Read the model definition and answer for the solid it produces. Units are mm, in the model's axes. A direction names the side the tool comes from. Coordinates: 2 decimals unless noted, no trailing zeros. Loops run counter-clockwise (first coordinate to the right, second up) from the corner with the lowest first, then second, coordinate; pieces in that order, holes last.
Autodesk Inventor part; units mm, degrees
ref_plane "YZ Plane" through (0, 0, 0) normal (1, 0, 0) x (0, 1, 0)
ref_plane "XZ Plane" through (0, 0, 0) normal (0, 1, 0) x (-1, 0, 0)
ref_plane "XY Plane" through (0, 0, 0) normal (0, 0, 1) x (1, 0, 0)
sketch "Sketch1" plane through (0, 0, 0) normal (1, 0, 0) x (0, 1, 0)
  point P0 (0, 0)
sketch "Sketch2" plane through (0, 0, 0) normal (1, 0, 0) x (0, 1, 0)
  line L0 (7, 8.85) -> (-7, 8.85)
  line L1 (-7, 8.85) -> (-7, -8.85)
  line L2 (-7, -8.85) -> (7, -8.85)
  line L3 (7, -8.85) -> (7, 8.85)
  point P0 (0, 0)
  dimension "d0" = 17.7
  dimension "d1" = 14
  dimension "d2" = 8.85
  dimension "d3" = 7
extrude "Extrusion1" add sketch "Sketch2" along normal blind 14
fillet "Fillet1" radius 2 2 edges at (7, 7, 8.85) (7, 7, -8.85)
sketch "Sketch5" plane through (14, 0, 0) normal (1, 0, 0) x (0, 0, -1)
  line L0 (-7.35, 6) -> (7.35, 6)
  line L1 (7.35, 6) -> (7.35, -7)
  line L2 (7.35, -7) -> (-7.35, -7)
  line L3 (-7.35, -7) -> (-7.35, 6)
  line L4 (6.85, 7) -> (-6.85, 7)
  line L5 (8.85, -7) -> (8.85, 5)
  line L6 (-8.85, -7) -> (8.85, -7)
  line L7 (-8.85, 5) -> (-8.85, -7)
  point P0 (0, 0)
  dimension "d19" = 1
  dimension "d20" = 1.5
  dimension "d21" = 0
  dimension "d22" = 1.5
extrude "Extrusion2" cut sketch "Sketch5" against normal blind 2
fillet "Fillet2" radius 1 1 edges at (13, 6, 7.35)
fillet "Fillet3" radius 1 1 edges at (13, 6, -7.35)
sketch "Sketch6" plane through (12, 0, 0) normal (1, 0, 0) x (0, 0, -1)
  line L0 (-3.75, 5.3) -> (3.75, 5.3)
  line L1 (3.75, 5.3) -> (3.75, -4.4)
  line L2 (3.75, -4.4) -> (-3.75, -4.4)
  line L3 (-3.75, -4.4) -> (-3.75, 5.3)
  line L4 (-6.35, 6) -> (6.35, 6)
  line L5 (7.35, -7) -> (-7.35, -7)
  line L6 (-7.35, -7) -> (-7.35, 5)
  line L7 (7.35, 5) -> (7.35, -7)
  point P0 (0, 0)
  dimension "d27" = 9.7
  dimension "d28" = 7.5
  dimension "d35" = 0.7
  dimension "d36" = 2.6
  dimension "d107" = 3.75
extrude "Extrusion3" cut sketch "Sketch6" against normal blind 2
ref_plane "Work Plane2" through (7, 0, 0) normal (1, 0, 0) x (0, 0, -1)
mirror "Mirror1" about plane through (7, 0, 0) normal (1, 0, 0) of "Extrusion2"
sketch "Sketch11" plane through (2, -7, -7.35) normal (-1, 0, 0) x (0, 0, 1)
  line L0 (4.45, 2) -> (10.25, 2)
  line L1 (10.25, 2) -> (10.25, 6.7)
  line L2 (10.25, 6.7) -> (4.45, 6.7)
  line L3 (4.45, 6.7) -> (4.45, 2)
  line L4 (10.725, 6.7) -> (3.975, 6.7)
  line L5 (3.975, 6.7) -> (3.975, 10)
  line L6 (3.975, 10) -> (10.725, 10)
  line L7 (10.725, 10) -> (10.725, 6.7)
  line L8 (14.7, 0) -> (0, 0)
  point P0 (7.35, 7)
  point P1 (10.25, 6.7)
  dimension "d52" = 5.8
  dimension "d53" = 4.7
  dimension "d54" = 2
  dimension "d55" = 3.3
  dimension "d56" = 6.75
  dimension "d57" = 2.9
  dimension "d58" = 3.375
extrude "Extrusion5" cut sketch "Sketch11" against normal blind 3.3
fillet "Fillet4" radius 0.001 2 edges at (3.65, 3, -3.375) (3.65, 3, 3.375)
fillet "Fillet5" radius 0.001 2 edges at (3.65, -0.3, -3.375) (3.65, -0.3, 3.375)
fillet "Fillet6" radius 1 1 edges at (1, 6, 7.35)
fillet "Fillet7" radius 1 1 edges at (1, 6, -7.35)
sketch "Sketch15" plane through (0, -7, -8.85) normal (0, -1, 0) x (1, 0, 0)
  line L0 (0, 2) -> (14, 2)
  circle A0 centre (4, 2) radius 0.5
  line L1 (0, 1.5) -> (0, 0)
  line L2 (12, 1.5) -> (12, 16.2)
  line L3 (2, 16.2) -> (2, 1.5)
  line L4 (7, 21.24) -> (7, -3.54)
  point P0 (0, 8.85)
  point P1 (12, 3.75)
  point P2 (2, 3.35)
  dimension "d74" = 1
  dimension "d120" = 4
extrude "Extrusion8" add sketch "Sketch15" along normal blind 4
mirror "Mirror3" about plane through (0, 0, 0) normal (0, 0, 1) of "Extrusion8"
mirror "Mirror4" about plane through (7, 0, 0) normal (1, 0, 0) of "Extrusion8", "Mirror3"
sketch "Sketch18" plane through (2, 3, -3.374) normal (0, -1, 0) x (1, 0, 0)
  line L0 (3.3, -0.001) -> (0, -0.001)
  line L1 (0, -0.001) -> (0, 6.749)
  line L2 (0, 6.749) -> (3.3, 6.749)
  line L3 (3.3, 6.749) -> (3.3, -0.001)
  line L4 (0, -0.001) -> (3.3, -0.001)
  line L5 (3.3, 6.749) -> (0, 6.749)
  line L6 (0, 0) -> (0, 6.748)
  line L7 (3.3, 0) -> (3.3, 6.748)
  point P0 (-2, 3.374)
extrude "Extrusion9" cut sketch "Sketch18" against normal through all
sketch "Sketch19" plane through (0, -7, 8.85) normal (0, -1, 0) x (1, 0, 0)
  line L0 (13, -0.8) -> (12, -0.8)
  line L1 (12, -0.8) -> (12, -1.5)
  line L2 (12, -1.5) -> (13, -1.5)
  line L3 (13, -1.5) -> (13, -0.8)
  point P0 (0, -8.85)
  dimension "d103" = 0.7
  dimension "d104" = 1
sketch3d "3D Sketch3"
  line L0 (14, -7, 7.35) -> (14, 5, 7.35)
  arc A0 (14, 5, 7.35) -> (14, 6, 6.35) centre (14, 5, 6.35) ccw
  line L1 (14, 6, 6.35) -> (14, 6, -6.35)
  arc A1 (14, 6, -6.35) -> (14, 5, -7.35) centre (14, 5, -6.35) ccw
  line L2 (14, 5, -7.35) -> (14, -7, -7.35)
sweep "Sweep3" cut profiles "Sketch19" path "3D Sketch3"
mirror "Mirror6" about plane through (7, 0, 0) normal (1, 0, 0) of "Sweep3"
sketch "Sketch20" plane through (12, 0, 0) normal (1, 0, 0) x (0, 0, -1)
  line L0 (-2.9, -5) -> (2.9, -5)
  line L1 (2.9, -5) -> (2.9, -7)
  line L2 (2.9, -7) -> (-2.9, -7)
  line L3 (-2.9, -7) -> (-2.9, -5)
  line L4 (3.6, 4.6) -> (3.6, -4.3)
  line L5 (-3.6, -4.3) -> (-3.6, 5.3)
  line L6 (3.6, -4.3) -> (-3.6, -4.3)
  line L7 (5.45, -7) -> (-5.45, -7)
  point P0 (0, 0)
  dimension "d109" = 0.7
  dimension "d110" = 0.7
  dimension "d116" = 2
extrude "Extrusion10" cut sketch "Sketch20" against normal through all
sketch "Sketch21" plane through (12, 0, 0) normal (1, 0, 0) x (0, 0, -1)
  line L0 (-2.9, -4.4) -> (2.9, -4.4)
  line L1 (2.9, -4.4) -> (2.9, -5)
  line L2 (2.9, -5) -> (-2.9, -5)
  line L3 (-2.9, -5) -> (-2.9, -4.4)
  line L4 (3.75, -4.4) -> (-3.75, -4.4)
  line L5 (-2.9, -5) -> (2.9, -5)
  line L6 (2.9, -5) -> (2.9, -7)
  line L7 (-2.9, -7) -> (-2.9, -5)
  point P0 (0, 0)
extrude "Extrusion11" cut sketch "Sketch21" against normal blind 2
properties part number "fingertip skeleton 5"
Item 1: Find the intervals of material crossed by line 1 along Y through (x, z) = (10.75, 3.5); line 2 along X through (y, z) = (6.25, -0.75); line 3 along X through (y, z) = (2, 8), in increasing order.
Numbers:
line 1: y = -7 to -4.4, 5.3 to 7
line 2: x = 0 to 1, 5.3 to 12, 13 to 14
line 3: x = 0 to 1, 2 to 12, 13 to 14
Item 2: Determine the mould class of faces 5 (the face through (3.892, -8.972, -6.362)), 6 (the face through (7, -1, -8.85)) for opening direction X: released by +X, released by -X, zero draft, split by the parting line, or undercut.
Numbers:
face 5: undercut
face 6: zero draft
Item 3: A cutting plane is placed at C-C on z = 4.75. Determine the outline of the cut face in (x, y), then the cut area to 3 significant figures.
Numbers:
outline: (0, 6) - (1, 6) - (1, 6.7) - (2, 6.7) - (2, -7) - (12, -7) - (12, 6.7) - (13, 6.7) - (13, 6) - (14, 6) - (14, 7) - (0, 7) - close
area: 143 mm2
Item 4: Which of the six approach directions +Z, -Z, +X, -X, +Y, -Y give full straight-line access (tool end or side, diameter ignored) to faces 1 (the face through (4, 5, 3.375)), 2 (the face through (13.493, 5.715, -7.049)), 3 (the face through (0.5, -1.1, -7.35)), 4 (the face through (11, 5.3, 0))?
Numbers:
face 1: +Y
face 2: +X, -Y
face 3: -X, -Y
face 4: +X
Item 5: Given pin 1 (1 mm diameter, centred on y = -3.5, z = -4, fed in from +X); pin 2 (2 mm diameter, centred on y = -0.5, z = -6, fed in from -X); pin 3 (4 mm diameter, centred on y = 1.5, z = 0, fed in from +X), each flat-ended and moving along its own axis, determine where each tip first touches the part or whether it passes through.
Numbers:
pin 1: stops at x = 12
pin 2: stops at x = 2
pin 3: stops at x = 10
Item 6: A cutting plane is placed at B-B on y = -6.5. Determine the outline of the cut face in (x, z).
Numbers:
outline: (0, -8.85) - (14, -8.85) - (14, -7.35) - (13, -7.35) - (13, -8.05) - (12, -8.05) - (12, -2.9) - (2, -2.9) - (2, -8.05) - (1, -8.05) - (1, -7.35) - (0, -7.35) - close; (0, 7.35) - (1, 7.35) - (1, 8.05) - (2, 8.05) - (2, 2.9) - (12, 2.9) - (12, 8.05) - (13, 8.05) - (13, 7.35) - (14, 7.35) - (14, 8.85) - (0, 8.85) - close
Item 7: A cutting plane is placed at D-D on y = -1. Determine the outline of the cut face in (x, z), then the cut area to 3 significant figures.
Numbers:
outline: (0, -8.85) - (14, -8.85) - (14, -7.35) - (13, -7.35) - (13, -8.05) - (12, -8.05) - (12, -3.75) - (10, -3.75) - (10, 3.75) - (12, 3.75) - (12, 8.05) - (13, 8.05) - (13, 7.35) - (14, 7.35) - (14, 8.85) - (0, 8.85) - (0, 7.35) - (1, 7.35) - (1, 8.05) - (2, 8.05) - (2, 2.9) - (5.3, 2.9) - (5.3, -2.9) - (2, -2.9) - (2, -8.05) - (1, -8.05) - (1, -7.35) - (0, -7.35) - close
area: 152 mm2
